Here's how the part is built. I have some questions about the finished solid (model axes, mm). Round coordinates to 2 decimals unless told otherwise and drop trailing zeros. Write each loop counter-clockwise with the first axis right and the second up, starting at its lowest first coordinate (ties: lowest second). Pieces come first, ordered by that corner, then holes. Notation, with made-up numbers: (38, 8) -> (79, 8) arc R12 ccw to (79, 13) -> close; hole circle Ø1 at (-9.5, 20.5). An arc over 180 degrees is marked (long way). Put each result on its own line as item: value. Start each with the question number.
1) I want a section at B-B, the plane z = 0. List the corners of the cut face in (x, y) for me.
2) If I drill on line 1 along Z through (x, y) = (35, 0); line 2 along Y through (x, z) = (63.5, -0.25); line 3 along Y through (x, z) = (27, -1.5), over which ranges is the centre line in solid material (lowest first)? Write a range as [from, to].
3) I want a section at A-A, the plane y = 0. List the corners of the cut face in (x, z) for me.
4) I want a section at C-C, the plane x = 84. List the corners of the cut face in (y, z) for me, then the cut area to 3 significant figures.
5) We'd pull the mould along Y, two halves only. Please class faces 1 (the flat face through (136, -1, -9)), 2 (the flat face through (67, 67.5, 0)), 3 (the cylindrical face through (67.048, 7.493, 0.33)): released by +Y, released by -Y, zero draft, split by the parting line, or undercut.
from build123d import *

# Parameters (mm, degrees)
F0_W     = 135
F0_H     = 20
F1_DEPTH = 136
F3_D     = 15


with BuildPart() as f1:
    # F0 (on Right) → F1 (new body)
    with BuildSketch(Plane.YZ):
        Rectangle(F0_W, F0_H)
    extrude(amount=F1_DEPTH)

    # F3 (through all)
    with Locations(Plane.YZ.offset(136)):
        with Locations((0, 0)):
            Hole(F3_D / 2)


solid = f1.part
Findings:
1. outline: (0, -67.5) -> (136, -67.5) -> (136, -7.5) -> (0, -7.5) -> close; (0, 7.5) -> (136, 7.5) -> (136, 67.5) -> (0, 67.5) -> close
2. line 1: z = [-10, -7.5], [7.5, 10]
2. line 2: y = [-67.5, -7.5], [7.5, 67.5]
2. line 3: y = [-67.5, -7.35], [7.35, 67.5]
3. outline: (0, -10) -> (136, -10) -> (136, -7.5) -> (0, -7.5) -> close; (0, 7.5) -> (136, 7.5) -> (136, 10) -> (0, 10) -> close
4. outline: (-67.5, -10) -> (67.5, -10) -> (67.5, 10) -> (-67.5, 10) -> close; hole circle Ø15 at (0, 0)
4. area: 2,520 mm2
5. face 1: zero draft
5. face 2: released by +Y
5. face 3: undercut
